Autodesk Inventor part; units mm, degrees
ref_plane "YZ Plane" through (0, 0, 0) normal (1, 0, 0) x (0, 1, 0)
ref_plane "XZ Plane" through (0, 0, 0) normal (0, 1, 0) x (-1, 0, 0)
ref_plane "XY Plane" through (0, 0, 0) normal (0, 0, 1) x (1, 0, 0)
sketch "Boceto1" plane through (0, 0, 0) normal (0, 0, 1) x (1, 0, 0)
  line L0 (-55.5895, 69.239) -> (57.1029, 69.239) construction
  line L1 (57.1029, 69.239) -> (57.1029, -41.5752) construction
  line L2 (57.1029, -41.5752) -> (-55.5895, -41.5752) construction
  line L3 (-55.5895, -41.5752) -> (-55.5895, 69.239) construction
  line L4 (-12.6216, 0) -> (12.6216, 0)
  line L5 (12.6216, 0) -> (12.6216, 3.1554)
  line L6 (12.6216, 3.1554) -> (22.7349, 3.1554)
  line L7 (22.7349, 3.1554) -> (22.7349, 26.032)
  arc A0 (22.7349, 26.032) -> (2.2249, 54.4304) centre (-2.0657, 29.7261) ccw
  arc A1 (2.2249, 54.4304) -> (-6.4524, 59.1635) centre (-6.058, 49.5659) ccw
  line L8 (-6.4524, 59.1635) -> (-4.8747, 53.6416)
  line L9 (-4.8747, 53.6416) -> (-11.1855, 50.4862)
  line L10 (-11.1855, 50.4862) -> (-12.7632, 45.7531)
  line L11 (-12.7632, 45.7531) -> (-23.8071, 37.8647)
  arc A2 (-23.8071, 37.8647) -> (-18.5481, 28.3985) centre (-17.1295, 35.3805) ccw
  line L12 (-18.5481, 28.3985) -> (-9.2432, 31.2863)
  line L13 (-9.2432, 31.2863) -> (-7.6971, 30.8036)
  line L14 (-7.6971, 30.8036) -> (-1.5746, 32.7037)
  arc A3 (-9.4662, 18.8123) -> (-1.5746, 32.7037) centre (-15.3564, 31.3458) ccw
  arc A4 (-9.4662, 18.8123) -> (-18.4064, 3.1554) centre (1.3548, 2.2525) ccw
  line L15 (-18.4064, 3.1554) -> (-12.6216, 3.1554)
  line L16 (-12.6216, 3.1554) -> (-12.6216, 0)
  line L17 (-18.5481, 28.3985) -> (-18.5481, 27.4104)
  line L18 (-18.5481, 27.4104) -> (-17.8555, 27.4104)
  line L19 (-17.8555, 27.4104) -> (-17.213, 28.8128)
  line L20 (-16.5658, 10.6295) -> (-16.5658, 13.4104)
  line L21 (-16.5658, 13.4104) -> (-15.3475, 12.8522)
  point P0 (0, 0)
  point P1 (-18.2018, 27.4104)
  dimension "d8" = 14
  dimension "d12" = 0.3463
extrude "Extrusión1" add sketch "Boceto1" along normal mid plane 10
properties part number "KIGTH TOP abrebotella medium 1.2"
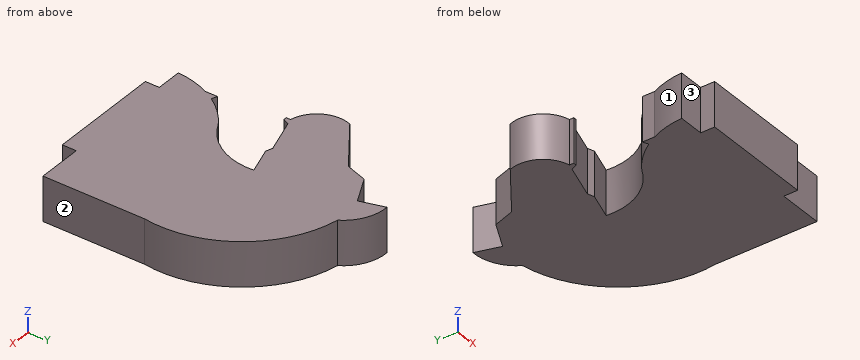
Geometry check sheet. Reference: the model listing, model coordinates, mm. Face numbers are marked on the shaded views. A direction names the side the tool comes from. Coordinates: 2 decimals unless noted, no trailing zeros. Order: outer loops, then holes, each group sorted by start corner. A loop starts at its lowest first (then second) coordinate and runs counter-clockwise, first axis right, second up. Notation, with made-up numbers: (42, 6.25) - (85, 6.25) arc R20 ccw to (85, 34.25) - close; hole circle Ø3 at (-13, -22.75). An arc over 180 degrees is marked (long way). Answer in a Markdown table with one row per item. Add a question column.
1. Section check D-D (x = 1). Enter the section's corners in (y, z).
2. Gauge pin test, flat ends, axial feed: pin 1 Ø5 at (y, z) = (17.5, 0.5) entering from +X; pin 2 Ø3 at (y, z) = (13.5, 0.5) entering from -X; pin 3 Ø1.6 at (y, z) = (1, -1) entering from -X. Record the tip position at first contact, or that the pin passes through.
3. Section check A-A (y = 32). Enter the section's corners in (x, z), plus the area to 3 significant figures.
4. Section check C-C (y = 16). Enter the section's corners in (x, z).
5. Section check B-B (z = -3). Enter the section's corners in (x, y).
6. Access from +Z, -Z, +X, -X, +Y, -Y to the whole of each face (thin tool, end or side, straight path). Record for the marked faces 1, 2 and 3.
7. Material ranges on L1, parallel to X at y = 11, z = 1; L2, parallel to Y at x = -3.5, z = -0.75; L3, parallel to Y at x = -7, z = 2.25, recorded low to high. Write a range as [from, to].
Data:
| question | item | result |
|---|---|---|
| 1 | outline | (0, -5) - (56.08, -5) - (56.08, 5) - (0, 5) - close |
| 2 | pin 1 | stops at x = 22.73 |
| 2 | pin 2 | stops at x = -16.57 |
| 2 | pin 3 | stops at x = -12.62 |
| 3 | outline | (-23.4, -5) - (-3.84, -5) - (-3.84, 5) - (-23.4, 5) - close; (-1.52, -5) - (22.91, -5) - (22.91, 5) - (-1.52, 5) - close |
| 3 | area | 440 mm² |
| 4 | outline | (-12.87, -5) - (22.73, -5) - (22.73, 5) - (-12.87, 5) - close |
| 5 | outline | (-23.81, 37.86) arc R7.12 ccw to (-18.55, 28.4) - (-18.55, 27.41) - (-17.86, 27.41) - (-17.21, 28.81) - (-9.24, 31.29) - (-7.7, 30.8) - (-1.57, 32.7) arc R13.85 cw to (-9.47, 18.81) arc R19.78 ccw to (-15.35, 12.85) - (-16.57, 13.41) - (-16.57, 10.63) arc R19.78 ccw to (-18.41, 3.16) - (-12.62, 3.16) - (-12.62, 0) - (12.62, 0) - (12.62, 3.16) - (22.73, 3.16) - (22.73, 26.03) arc R25.07 ccw to (2.22, 54.43) arc R9.61 ccw to (-6.45, 59.16) - (-4.87, 53.64) - (-11.19, 50.49) - (-12.76, 45.75) - close |
| 6 | face 1 | +Z, -Z, -X |
| 6 | face 2 | +Z, -Z, +X, -Y |
| 6 | face 3 | +Z, -Z, -X, -Y |
| 7 | L1 | x = [-16.57, 22.73] |
| 7 | L2 | y = [0, 24.19], [32.11, 58.82] |
| 7 | L3 | y = [0, 20.3], [31.02, 52.58] |
